Work out the finished part from the listing and answer in its coordinate system (mm). Face numbers are marked on the shaded views. Round coordinates to 2 decimals unless told otherwise and drop trailing zeros. Loops run counter-clockwise (first coordinate to the right, second up) from the corner with the lowest first, then second, coordinate; pieces in that order, holes last. Notation, with made-up numbers: (-0.5, -4) -> (17.5, -4) arc R15 cw to (17.5, 4) -> close; hole circle Ø1 at (21.25, -12.5). An arc over 180 degrees is marked (long way). Use one line per item in the form item = value.
```python
from build123d import *
from build123d.topology import SkipClean

# Parameters (mm, degrees)
BOSS_EXTRUDE1_DEPTH = 1.5
SKETCH2_R           = 4
BOSS_EXTRUDE2_DEPTH = 2.5
BOSS_EXTRUDE3_START = 0.8
SKETCH3_R           = 4
BOSS_EXTRUDE3_DEPTH = 0.8
SKETCH4_R           = 1.5
CUT_EXTRUDE1_DEPTH  = 16.697133496


with BuildPart() as part:
    # Sketch1 → Boss-Extrude1 (new body)
    with BuildSketch(Plane.XY):
        with BuildLine():
            Line((-1.892714844, 12.666224303), (-2.75, 2.90473751))
            ThreePointArc((-2.75, 2.90473751), (-4, 0), (-2.75, -2.90473751))
            Line((-2.75, -2.90473751), (-1.892714844, -12.666224303))
            ThreePointArc((-1.892714844, -12.666224303), (0, -14.4), (1.892714844, -12.666224303))
            Line((1.892714844, -12.666224303), (2.75, -2.90473751))
            ThreePointArc((2.75, -2.90473751), (4, 0), (2.75, 2.90473751))
            Line((2.75, 2.90473751), (1.892714844, 12.666224303))
            ThreePointArc((1.892714844, 12.666224303), (0, 14.4), (-1.892714844, 12.666224303))
        make_face()
    extrude(amount=BOSS_EXTRUDE1_DEPTH)

    # Sketch2 → Boss-Extrude2 (add)
    with BuildSketch(Plane.XY.offset(1.5)):
        with Locations(Location((0, 0, 0), (0, 0, 226.567463442))):
            Circle(SKETCH2_R)
    extrude(amount=BOSS_EXTRUDE2_DEPTH)

    # Sketch3 → Boss-Extrude3 (add)
    with SkipClean():  # the faces are left unmerged after this step: merging them gives an invalid solid
        with BuildSketch(Plane(origin=(0, 0, 0), x_dir=(-1, 0, 0), z_dir=(0, 0, -1)).offset(BOSS_EXTRUDE3_START)):
            Circle(SKETCH3_R)
        extrude(amount=-BOSS_EXTRUDE3_DEPTH)
    add(part.part.scale(1), mode=Mode.REPLACE)  # the faces are merged on a copy

    # Sketch4 → Cut-Extrude1 (cut, through all)
    with BuildSketch(Plane(origin=(0, 0, -0.8), x_dir=(-1, 0, 0), z_dir=(0, 0, -1))):
        Circle(SKETCH4_R)
    extrude(amount=-CUT_EXTRUDE1_DEPTH, mode=Mode.SUBTRACT)


solid = part.part
```
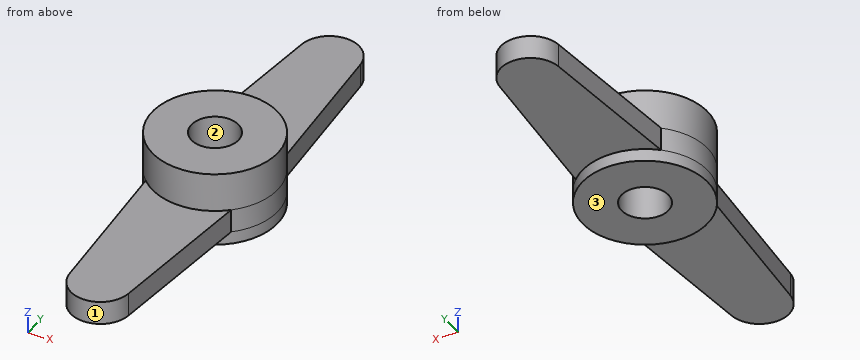
(1) Find section A-A, the plane y = 0. Write down the section's boundary in (x, z).
Completed:
outline = (-4, -0.8) -> (-1.5, -0.8) -> (-1.5, 4) -> (-4, 4) -> close; (1.5, -0.8) -> (4, -0.8) -> (4, 4) -> (1.5, 4) -> close
(2) Find section D-D, the plane x = 3. Write down the section's boundary in (y, z).
Completed:
outline = (-2.65, -0.8) -> (2.65, -0.8) -> (2.65, 4) -> (-2.65, 4) -> close
(3) Consider L1, parallel to Y at x = 0, z = 0.3; L2, parallel to Z at x = -1, y = -4.25; L3, parallel to Y at x = -2.75, z = 1.5. Determine where each line is inside the solid, lowest interval first.
Completed:
L1 = -14.4 to -1.5, 1.5 to 14.4
L2 = 0 to 1.5
L3 = -2.9 to 2.9
(4) For a pull along X with two mould halves and no side action, classify the marked faces 1, 2 and 3 as +X half, -X half, draft (parallel to the pull), parting line (faces both ways), or undercut.
Completed:
face_1 = parting line
face_2 = undercut
face_3 = draft
(5) Find section B-B, the plane z = 0.95. Write down the section's boundary in (x, y), then the cut area to 3 significant figures.
Completed:
outline = (-2.75, -2.9) -> (-1.89, -12.67) arc R1.9 ccw to (1.89, -12.67) -> (2.75, -2.9) arc R4 ccw to (2.75, 2.9) -> (1.89, 12.67) arc R1.9 ccw to (-1.89, 12.67) -> (-2.75, 2.9) arc R4 ccw to start; hole circle Ø3 at (0, 0)
area = 136 mm2
(6) Find section C-C, the plane x = 0. Write down the section's boundary in (y, z), then the cut area to 3 significant figures.
Completed:
outline = (-14.4, 0) -> (-4, 0) -> (-4, -0.8) -> (-1.5, -0.8) -> (-1.5, 4) -> (-4, 4) -> (-4, 1.5) -> (-14.4, 1.5) -> close; (1.5, -0.8) -> (4, -0.8) -> (4, 0) -> (14.4, 0) -> (14.4, 1.5) -> (4, 1.5) -> (4, 4) -> (1.5, 4) -> close
area = 55.2 mm2
(7) Given P1, Ø1.5, axis at y = -1.5, z = 2.5, coming from the -X side; P2, Ø1.6, axis at x = 1, y = 7.5, coming from the +Z side; P3, Ø4.5, axis at x = 0, y = 9, coming from the -Z side, each flat-ended and moving along its own axis, determine where each tip first touches the part or whether it passes through.
Completed:
P1 = -3.93
P2 = 1.5
P3 = 0
